Can you work these out from the drawing? Everything is in mm from the part's minimum corner. A direction names the side the tool comes from. Give positions to 0.01 mm unless a question says otherwise; leave off trailing zeros. Write each loop counter-clockwise with the first axis right and the second up, starting at its lowest first coordinate (ties: lowest second). Pieces come first, ordered by that corner, then holes. Notation, with made-up numbers: M 3.5,4 L 59.5,4 A26 ccw 59.5,21 Z; hole C 62.5,-15.75 d2. An arc over 180 degrees is marked long. One line per item, written item: value.
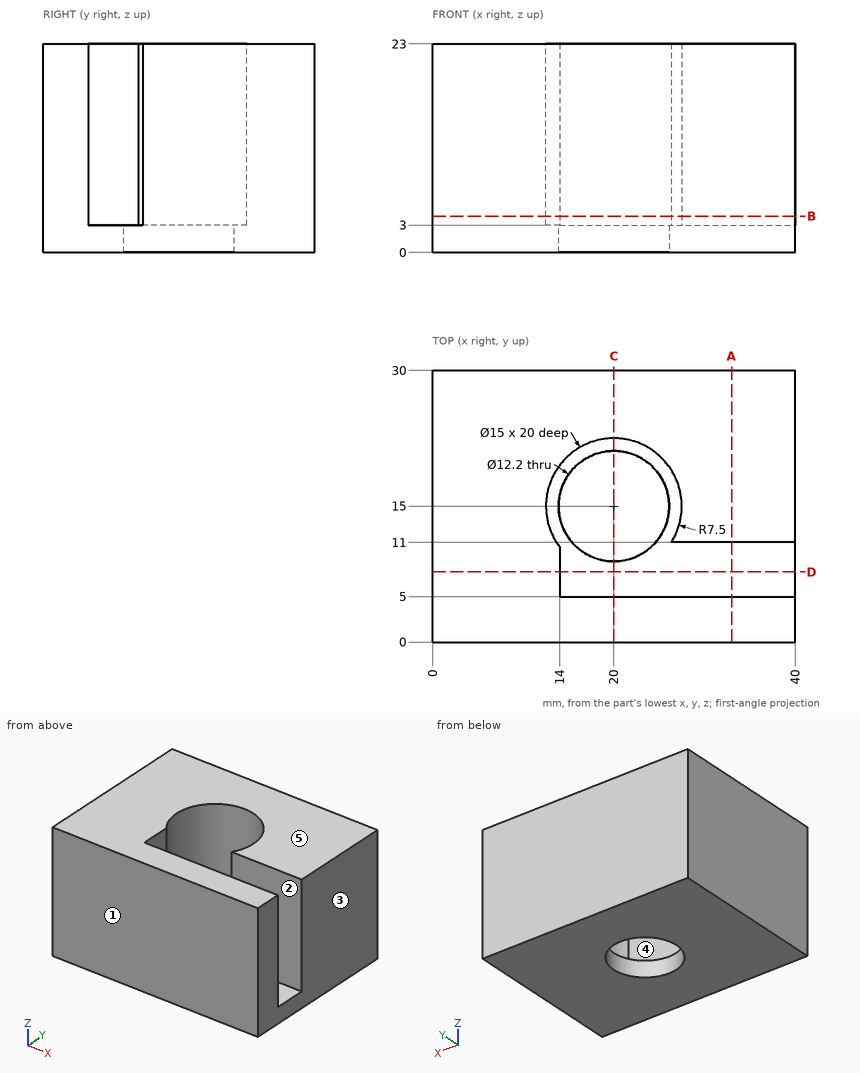
1) On a 3-axis mill with a long thin cutter (end or side, diameter ignored), from which of +Z, -Z, +X, -X, +Y, -Y can I reach the whole of each face in a straight line? I mean the marked faces 4 and 5. Say none if no direction works.
Outcome:
face 4: +Z, +X
face 5: +Z, +X, -X, +Y, -Y
2) If we section it at D-D, the plane y = 7.75: Write out the boundary of the cut face in (x, z).
Outcome:
outline: M 0,0 L 40,0 L 40,3 L 14,3 L 14,23 L 0,23 Z
3) If we section it at A-A, the plane x = 33: Write out the boundary of the cut face in (y, z).
Outcome:
outline: M 0,0 L 30,0 L 30,23 L 11,23 L 11,3 L 5,3 L 5,23 L 0,23 Z
4) If we section it at B-B, the plane z = 4: Write out the boundary of the cut face in (x, y).
Outcome:
outline: M 0,0 L 40,0 L 40,5 L 14,5 L 14,10.5 A7.5 cw long 26.34,11 L 40,11 L 40,30 L 0,30 Z
5) We'd pull the mould along Y, two halves only. Please class the marked faces 1, 2 and 3: pulls with the +Y half, pulls with the -Y half, needs draft (parallel to the pull), parting line crosses it, or undercut.
Outcome:
face 1: pulls with the -Y half
face 2: undercut
face 3: needs draft
6) Please list where these lines run through material, in increasing order: L1, parallel to Y at x = 20, z = 1; L2, parallel to X at y = 15, z = 13.5; L3, parallel to Z at x = 14, y = 13. Write a range as from..to.
Outcome:
L1: y = 0..8.9, 21.1..30
L2: x = 0..12.5, 27.5..40
L3: z = 0..3
7) If we section it at C-C, the plane x = 20: Write out the boundary of the cut face in (y, z), then the cut area to 3 significant figures.
Outcome:
outline: M 0,0 L 8.9,0 L 8.9,3 L 5,3 L 5,23 L 0,23 Z; M 21.1,0 L 30,0 L 30,23 L 22.5,23 L 22.5,3 L 21.1,3 Z
area: 303 mm^2
